```python
from build123d import *

# Parameters (mm, degrees)
SKIZZE1_R                       = 2
AUFSATZ_LINEAR_AUSTRAGEN1_DEPTH = 75
SKIZZE7_W                       = 0.9
SKIZZE7_H                       = 0.25
SCHNITT_LINEAR_AUSTRAGEN1_DEPTH = 27


with BuildPart() as part:
    # Skizze1 → Aufsatz-Linear austragen1 (new, symmetric)
    with BuildSketch(Plane.XY):
        Circle(SKIZZE1_R)
    extrude(amount=AUFSATZ_LINEAR_AUSTRAGEN1_DEPTH, both=True)

    # Skizze7 → Schnitt-Rotation1 (revolve, cut)
    with BuildSketch(Plane(origin=(0, 0, 0), x_dir=(0, 0, -1), z_dir=(1, 0, 0))):
        with Locations((-72.75, 1.875)):
            Rectangle(SKIZZE7_W, SKIZZE7_H)
        with Locations((48.65, 1.875)):
            Rectangle(SKIZZE7_W, SKIZZE7_H)
    revolve(axis=Axis((0, 0, -75), (0, 0, 1)), mode=Mode.SUBTRACT)

    # Skizze8 → Schnitt-Linear austragen1 (cut)
    with BuildSketch(Plane.XY.offset(75)):
        with BuildLine():
            Line((1.2, 1.6), (-1.2, 1.6))
            ThreePointArc((-1.2, 1.6), (0, 2), (1.2, 1.6))
        make_face()
    extrude(amount=-SCHNITT_LINEAR_AUSTRAGEN1_DEPTH, mode=Mode.SUBTRACT)


solid = part.part
```
Geometry check sheet. Reference: the model listing, model coordinates, mm. A direction names the side the tool comes from. Round coordinates to 2 decimals unless told otherwise and drop trailing zeros. Order: outer loops, then holes, each group sorted by start corner. A loop starts at its lowest first (then second) coordinate and runs counter-clockwise, first axis right, second up. Notation, with made-up numbers: (81.5, 64) - (117.5, 64) arc R23 cw to (117.5, 91) - close; hole circle Ø5 at (-13, 40.5). An arc over 180 degrees is marked (long way). Use a Markdown table: item, result. Add a question column.
(1) Sectioned sample at B-B, the plane z = -4.5. Enter the section's corners in (x, y), and give its area (3 significant figures).
(2) Sectioned sample at A-A, the plane x = 0. Enter the section's corners in (y, z), and give its area (3 significant figures).
(3) Material ranges on line 1 along Y through (x, z) = (0.25, -56.5); line 2 along Z through (x, y) = (0.6, 1.8); line 3 along Y through (x, z) = (1.1, 39.5), recorded low to high. Write a range as [from, to].
(4) Depth check by flat-ended pin: pin 1 (0.7 mm diameter, centred on x = 0.5, z = 63, fed in from +Y). Enter the tip coordinate at first touch or a pass-through.
(5) Tool access check on faces 4 (the flat face through (0, 1.6, 62)), 5 (the cylindrical face through (-0.07, -1.75, 72.74)), 6 (the cylindrical face through (1.847, -0.766, -61.869)). Record the directions out of +Z, -Z, +X, -X, +Y, -Y that give a thin tool (end or side, any length) a straight path to the whole face; none if there is none.
(6) Release check for a two-part mould opening along Z. For faces 1 (the flat face through (0, 0, -75)), 2 (the flat face through (0, 0, 75)), 3 (the cylindrical face through (0.67, 1.617, -48.656)) record: pulls with the +Z half, pulls with the -Z half, needs draft (parallel to the pull), parting line crosses it, or undercut.
Answers below:
| question | item | result |
|---|---|---|
| 1 | outline | circle Ø4 at (0, 0) |
| 1 | area | 12.6 mm² |
| 2 | outline | (-2, -75) - (2, -75) - (2, -49.1) - (1.75, -49.1) - (1.75, -48.2) - (2, -48.2) - (2, 48) - (1.6, 48) - (1.6, 75) - (-2, 75) - (-2, 73.2) - (-1.75, 73.2) - (-1.75, 72.3) - (-2, 72.3) - (-2, -48.2) - (-1.75, -48.2) - (-1.75, -49.1) - (-2, -49.1) - close |
| 2 | area | 589 mm² |
| 3 | line 1 | [-1.98, 1.98] |
| 3 | line 2 | [-75, -49.1], [-48.2, 48] |
| 3 | line 3 | [-1.67, 1.67] |
| 4 | pin 1 | y = 1.6 |
| 5 | face 4 | +Z, +X, -X, +Y |
| 5 | face 5 | none |
| 5 | face 6 | +Z, -Z |
| 6 | face 1 | pulls with the -Z half |
| 6 | face 2 | pulls with the +Z half |
| 6 | face 3 | undercut |
